Design review of the part built by this model. Coordinates are the model's own, in mm. A direction names the side the tool comes from. Round coordinates to 2 decimals unless told otherwise and drop trailing zeros. Loops run counter-clockwise (first coordinate to the right, second up) from the corner with the lowest first, then second, coordinate; pieces in that order, holes last. Notation, with made-up numbers: (84, 34.5) -> (114, 34.5) arc R24 ccw to (114, 47.5) -> close; hole circle Ø1 at (58, -24). An arc over 180 degrees is marked (long way). Answer as CSV lines item,"result". Start each with the question number.
(1) Draft analysis for pull direction Y (two halves, no side actions). For faces 3 (the face through (24.614, 21.128, 55.07)), 4 (the face through (19.7, 19.8, 0)), 5 (the face through (20, 50, 55)), state which applies: +Y half, -Y half, draft (parallel to the pull), parting line (faces both ways), or undercut.
(2) Machinability: for faces 1 (the face through (15, 10, 39)), 2 (the face through (40, 8, 30)), which of the approach directions +Z, -Z, +X, -X, +Y, -Y give a long, thin tool a straight path to every point of the face, cutting with its end or side? Answer none if there is none.
(3) To check wall thickness, follow line 1 (Z direction, x = 35.5, y = 33); line 2 (Y direction, x = 20, z = 56); line 3 (X direction, y = 5, z = 30). State the ranges of each line that lie inside material, in increasing order. Write a range as from..to.
(4) Take a section at D-D, the plane y = 31.5. Write out the cut boundary in (x, z).
(5) Take a section at A-A, the plane y = 17. Write out the cut boundary in (x, z), and give its area (3 significant figures).
(6) Take a section at B-B, the plane x = 20. Write out the cut boundary in (y, z).
(7) Take a section at C-C, the plane z = 30. Write out the cut boundary in (x, y), and give its area (3 significant figures).
from build123d import *

# Parameters (mm, degrees)
SKETCH1_W           = 40
SKETCH1_H           = 10
BOSS_EXTRUDE1_DEPTH = 30
SKETCH1_3_R         = 10
BOSS_EXTRUDE2_DEPTH = 10
SKETCH3_R           = 10
CUT_EXTRUDE1_DEPTH  = 10


with BuildPart() as part:
    # Sketch1 → Boss-Extrude1 (new body)
    with BuildSketch(Plane.XY):
        with Locations((20, 5)):
            Rectangle(SKETCH1_W, SKETCH1_H)
    boss_extrude1 = extrude(amount=BOSS_EXTRUDE1_DEPTH)

    # Sketch1_3 → Boss-Extrude2 (add)
    with BuildSketch(Plane.XY):
        with BuildLine():
            Line((0, 30), (0, 10))
            Line((0, 10), (40, 10))
            Line((40, 10), (40, 30))
            ThreePointArc((40, 30), (20, 50), (0, 30))
        make_face()
        with Locations((20, 30)):
            Circle(SKETCH1_3_R, mode=Mode.SUBTRACT)
    boss_extrude2 = extrude(amount=BOSS_EXTRUDE2_DEPTH)

    # Mirror2: Boss-Extrude1, Boss-Extrude2 across plane
    add(boss_extrude1.mirror(Plane.XY.offset(30)))
    add(boss_extrude2.mirror(Plane.XY.offset(30)))

    # Sketch3 → Cut-Extrude1 (cut)
    with BuildSketch(Plane(origin=(0, 0, 0), x_dir=(1, 0, 0), z_dir=(0, 1, 0))):
        with Locations(Location((20, -30, 0), (0, 0, 270))):
            Circle(SKETCH3_R)
    extrude(amount=CUT_EXTRUDE1_DEPTH, mode=Mode.SUBTRACT)


solid = part.part
The answers:
1,face 3,"undercut"
1,face 4,"draft"
1,face 5,"+Y half"
2,face 1,"+X, -X, +Y"
2,face 2,"+Z, -Z, +X, +Y, -Y"
3,line 1,"0..10, 50..60"
3,line 2,"0..20, 40..50"
3,line 3,"0..10, 30..40"
4,outline,"(0.06, 0) -> (10.11, 0) -> (10.11, 10) -> (0.06, 10) -> close; (0.06, 50) -> (10.11, 50) -> (10.11, 60) -> (0.06, 60) -> close; (29.89, 0) -> (39.94, 0) -> (39.94, 10) -> (29.89, 10) -> close; (29.89, 50) -> (39.94, 50) -> (39.94, 60) -> (29.89, 60) -> close"
5,outline,"(0, 0) -> (40, 0) -> (40, 10) -> (0, 10) -> close; (0, 50) -> (40, 50) -> (40, 60) -> (0, 60) -> close"
5,area,"800 mm²"
6,outline,"(0, 0) -> (20, 0) -> (20, 10) -> (10, 10) -> (10, 20) -> (0, 20) -> close; (0, 40) -> (10, 40) -> (10, 50) -> (20, 50) -> (20, 60) -> (0, 60) -> close; (40, 0) -> (50, 0) -> (50, 10) -> (40, 10) -> close; (40, 50) -> (50, 50) -> (50, 60) -> (40, 60) -> close"
7,outline,"(0, 0) -> (10, 0) -> (10, 10) -> (0, 10) -> close; (30, 0) -> (40, 0) -> (40, 10) -> (30, 10) -> close"
7,area,"200 mm²"
